Print and shaded views of the part. All mm, measured from the part's lowest x, y and z. Round coordinates to 2 decimals unless told otherwise and drop trailing zeros. Order: outer loops, then holes, each group sorted by start corner. A loop starts at its lowest first (then second) coordinate and runs counter-clockwise, first axis right, second up. Notation, with made-up numbers: M 80.25,-29.75 L 139.25,-29.75 A19 ccw 139.25,-12.75 Z; hole C 7,-14 d9. An arc over 180 degrees is marked long. Write each question's results on one line, items separated by ' | '. Start each with the question number.
1. Band-saw the part on A-A, the plane y = 18. List the corners of the cut face in (x, z).
2. Band-saw the part on B-B, the plane z = 306. List the corners of the cut face in (x, y).
3. Drop flat-ended pins along their axis: pin 1 Ø7 at (x, y) = (28, 21.5) entering from -Z; pin 2 Ø2 at (x, z) = (400.5, 340.5) entering from -Y; pin 3 Ø7 at (x, y) = (616, 12) entering from +Z; pin 4 Ø5 at (x, y) = (319, 36) entering from -Z. Give the stop position or say it passes through.
4. Band-saw the part on C-C, the plane z = 210. List the corners of the cut face in (x, y), then the cut area to 3 significant figures.
5. Band-saw the part on D-D, the plane x = 105. List the corners of the cut face in (y, z).
6. Probe L1, parallel to Y at x = 513, z = 350; L2, parallel to X at y = 6, z = 273; L3, parallel to Z at x = 29, y = 2. List the from-to ranges inside material, lowest first. Write a range as [from, to].
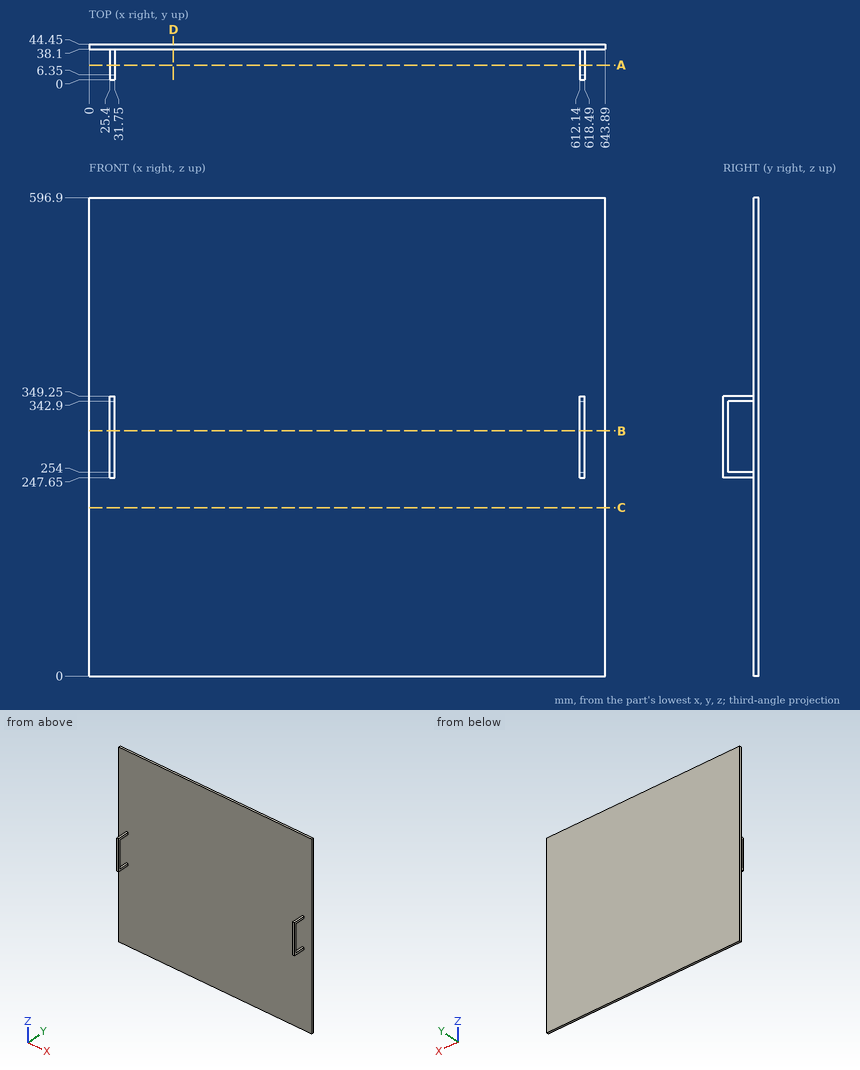
Solution:
1) outline: M 25.4,247.65 L 31.75,247.65 L 31.75,254 L 25.4,254 Z; M 25.4,342.9 L 31.75,342.9 L 31.75,349.25 L 25.4,349.25 Z; M 612.14,247.65 L 618.49,247.65 L 618.49,254 L 612.14,254 Z; M 612.14,342.9 L 618.49,342.9 L 618.49,349.25 L 612.14,349.25 Z
2) outline: M 0,38.1 L 643.89,38.1 L 643.89,44.45 L 0,44.45 Z; M 25.4,0 L 31.75,0 L 31.75,6.35 L 25.4,6.35 Z; M 612.14,0 L 618.49,0 L 618.49,6.35 L 612.14,6.35 Z
3) pin 1: z = 247.65 | pin 2: y = 38.1 | pin 3: z = 349.25 | pin 4: z = 0
4) outline: M 0,38.1 L 643.89,38.1 L 643.89,44.45 L 0,44.45 Z | area: 4,090 mm^2
5) outline: M 38.1,0 L 44.45,0 L 44.45,596.9 L 38.1,596.9 Z
6) L1: [38.1, 44.45] | L2: [25.4, 31.75], [612.14, 618.49] | L3: [247.65, 349.25]
